Check sheet for the modelled part. Datum: model origin and axes. Units: mm. Coordinates: 2 decimals unless noted, no trailing zeros. Loops run counter-clockwise (first coordinate to the right, second up) from the corner with the lowest first, then second, coordinate; pieces in that order, holes last. Notation, with made-up numbers: (43.25, 22.5) -> (97.25, 22.5) arc R27 cw to (97.25, 39.5) -> close; hole circle Ø9 at (33, 51). An arc over 180 degrees is marked (long way). Use one line per item in the form item = value.
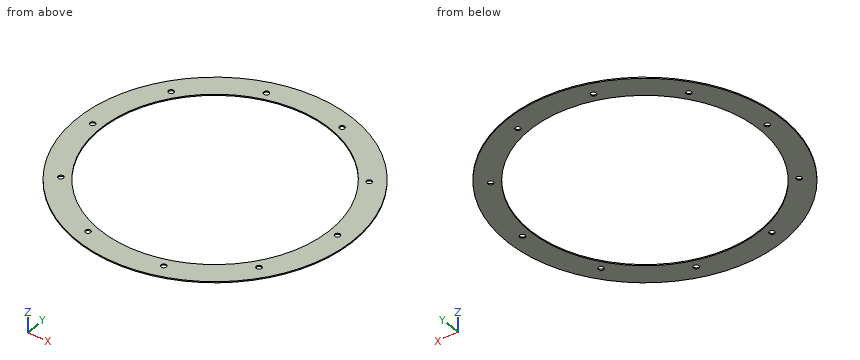
Autodesk Inventor part; units mm, degrees
ref_plane "Work Plane1" through (0, 0, 0) normal (0, 0, 1) x (1, 0, 0)
ref_plane "YZ Plane" through (0, 0, 0) normal (1, 0, 0) x (0, 1, 0)
ref_plane "XZ Plane" through (0, 0, 0) normal (0, 1, 0) x (-1, 0, 0)
ref_plane "Work Plane1" through (0, 0, 0) normal (0, 0, 1) x (1, 0, 0)
sketch "Sketch1" plane through (0, 0, 0) normal (0, 0, 1) x (1, 0, 0)
  circle A0 centre (26.4627, -50.6671) radius 1.8415
  circle A1 centre (69.5627, -81.9811) radius 1.8415
  circle A2 centre (122.8373, -81.9811) radius 1.8415
  circle A3 centre (165.9373, -50.6671) radius 1.8415
  circle A4 centre (182.4, 0) radius 1.8415
  circle A5 centre (165.9373, 50.6671) radius 1.8415
  circle A6 centre (122.8373, 81.9811) radius 1.8415
  circle A7 centre (69.5627, 81.9811) radius 1.8415
  circle A8 centre (26.4627, 50.6671) radius 1.8415
  circle A9 centre (10, 0) radius 1.8415
  circle A10 centre (96.2, 0) radius 80.1116
  circle A11 centre (96.2, 0) radius 96.2
  point P0 (0, 0)
extrude "Extrusion1" add sketch "Sketch1" along normal blind 0.7937
properties part number "1139_Outer Gasket_V1" material "Rubber"
(1) Go/stop test with a flat-tipped pin: P1, Ø3.5, axis at x = 122.84, y = -81.98, coming from the +Z side. Record where the tip stops, or that it passes through.
Established:
P1 = through
(2) Section check C-C, the plane z = 0.5. Give the number of separate pieces and of enclosed holes in the cut face, plus the area to 3 significant figures.
Established:
separate_pieces = 1
enclosed_holes = 11
area = 8,800 mm²
(3) Section check A-A, the plane x = 96.2. Record the boundary of the cut face in (y, z).
Established:
outline = (-96.2, 0) -> (-80.11, 0) -> (-80.11, 0.79) -> (-96.2, 0.79) -> close; (80.11, 0) -> (96.2, 0) -> (96.2, 0.79) -> (80.11, 0.79) -> close
(4) Scan lines: line 1 along X through (y, z) = (1, 0.35); line 2 along Y through (x, z) = (164.5, 0.25); line 3 along Y through (x, z) = (126, 0.2). Record each from-to range of solid material in increasing order.
Established:
line_1 = 0.01 to 8.45, 11.55 to 16.09, 176.31 to 180.85, 183.95 to 192.39
line_2 = -67.75 to -51.82, -49.52 to -41.87, 41.87 to 49.52, 51.82 to 67.75
line_3 = -91.47 to -74.36, 74.36 to 91.47
(5) Section check B-B, the plane y = -43.5. Record the boundary of the cut face in (x, z), plus the area to 3 significant figures.
Established:
outline = (10.4, 0) -> (28.93, 0) -> (28.93, 0.79) -> (10.4, 0.79) -> close; (163.47, 0) -> (182, 0) -> (182, 0.79) -> (163.47, 0.79) -> close
area = 29.4 mm²
